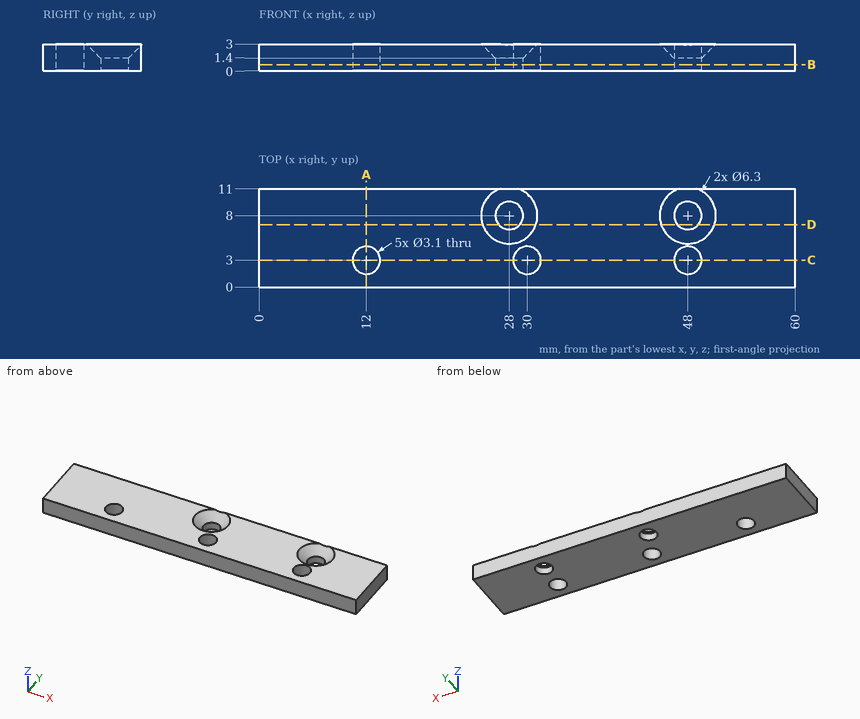
Input: dimensioned drawing with shaded views. Units: mm. Origin: part minimum x, y, z. Give positions to 0.01 mm unless a question says otherwise; leave off trailing zeros. Loops run counter-clockwise (first coordinate to the right, second up) from the corner with the lowest first, then second, coordinate; pieces in that order, holes last. Notation, with made-up numbers: (1, 87.25) -> (30, 87.25) arc R37 cw to (30, 123.25) -> close; hole circle Ø9 at (23.5, -24.75). An arc over 180 degrees is marked (long way). Use a Markdown table: item, result. Add a question column.
1) Section query C-C, the plane y = 3. Return the cut outline in (x, z), then the cut area to 3 significant figures.
2) Section query D-D, the plane y = 7. Count the separate pieces of the cut face and the enclosed holes in it, then the cut area to 3 significant figures.
3) Section query A-A, the plane x = 12. Return the cut outline in (y, z).
4) First-contact query: pin 1 (4 mm diameter, centred on x = 48, y = 8, fed in from +Z); pin 2 (3 mm diameter, centred on x = 28, y = 8, fed in from +Z). Flat tips, straight axial feed; report the tip coordinate or a pass-through.
5) Line query: line 1 along Y through (x, z) = (48, 0.7); line 2 along X through (y, z) = (9.25, 2.85); line 3 along X through (y, z) = (5.75, 2.8). Output: solid intervals per line, ascending. Write a range as [from, to].
6) Section query B-B, the plane z = 0.7. Return the cut outline in (x, y).
Numbers:
| question | item | result |
|---|---|---|
| 1 | outline | (0, 0) -> (10.45, 0) -> (10.45, 3) -> (0, 3) -> close; (13.55, 0) -> (28.45, 0) -> (28.45, 3) -> (13.55, 3) -> close; (31.55, 0) -> (46.45, 0) -> (46.45, 3) -> (31.55, 3) -> close; (49.55, 0) -> (60, 0) -> (60, 3) -> (49.55, 3) -> close |
| 1 | area | 152 mm2 |
| 2 | separate pieces | 3 |
| 2 | enclosed holes | 0 |
| 2 | area | 160 mm2 |
| 3 | outline | (0, 0) -> (1.45, 0) -> (1.45, 3) -> (0, 3) -> close; (4.55, 0) -> (11, 0) -> (11, 3) -> (4.55, 3) -> close |
| 4 | pin 1 | stops at z = 1.85 |
| 4 | pin 2 | passes through |
| 5 | line 1 | y = [0, 1.45], [4.55, 6.45], [9.55, 11] |
| 5 | line 2 | x = [0, 25.27], [30.73, 45.27], [50.73, 60] |
| 5 | line 3 | x = [0, 26.09], [29.91, 46.09], [49.91, 60] |
| 6 | outline | (0, 0) -> (60, 0) -> (60, 11) -> (0, 11) -> close; hole circle Ø3.1 at (12, 3); hole circle Ø3.1 at (28, 8); hole circle Ø3.1 at (30, 3); hole circle Ø3.1 at (48, 3); hole circle Ø3.1 at (48, 8) |
